The figure shows three views and two pictorial views of one solid part (mm, origin at its lowest corner). Answer the questions. A direction names the side the tool comes from. Round coordinates to 2 decimals unless told otherwise and drop trailing zeros. Write each loop counter-clockwise with the first axis right and the second up, starting at its lowest first coordinate (ties: lowest second). Pieces come first, ordered by that corner, then holes.
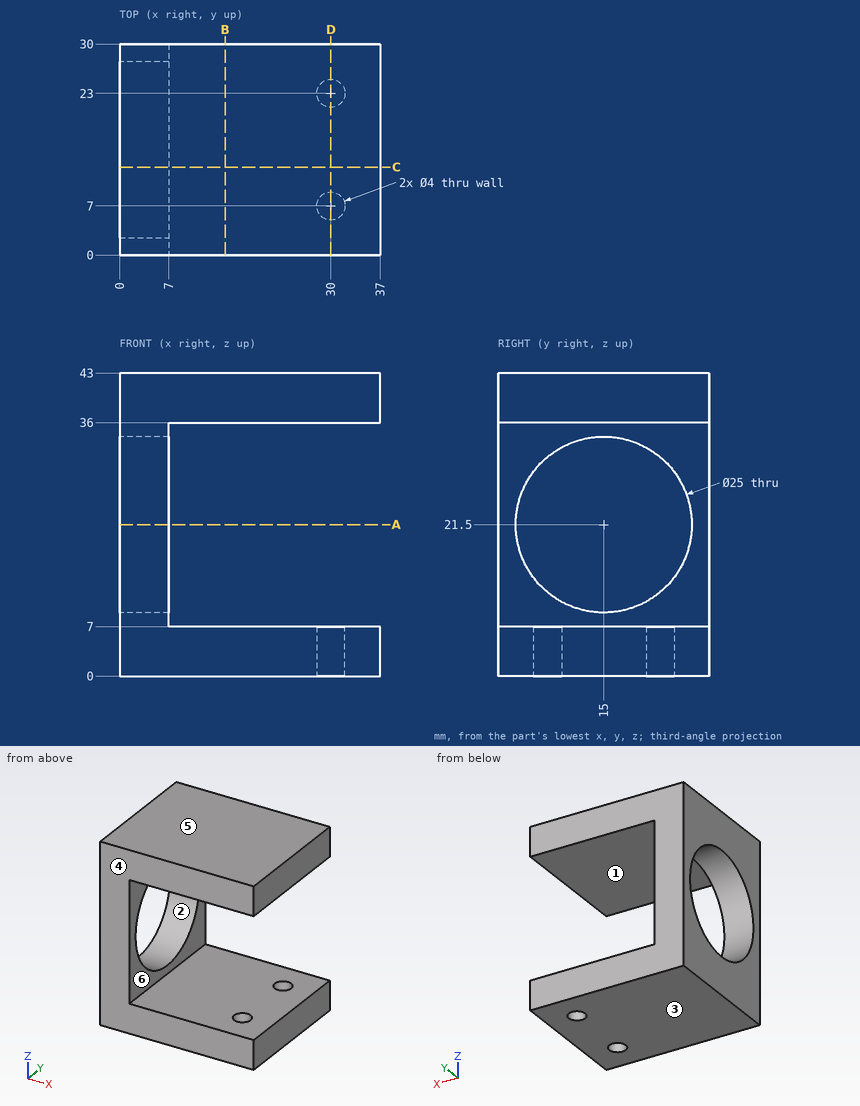
Q1. Straight lines are drawn through the part: probe 1 along Y at (x, z) = (30, 2.75); probe 2 along Z at (x, y) = (21, 18.25); probe 3 along X at (y, z) = (7, 5). For each, find the intervals that lie inside material, in ascending order.
Verdict:
probe 1: y = 0 to 5, 9 to 21, 25 to 30
probe 2: z = 0 to 7, 36 to 43
probe 3: x = 0 to 28, 32 to 37
Q2. Section A-A (z = 21.5) is taken. Determine the outline of the cut face in (x, y), then the cut area to 3 significant figures.
Verdict:
outline: (0, 0) - (7, 0) - (7, 2.5) - (0, 2.5) - close; (0, 27.5) - (7, 27.5) - (7, 30) - (0, 30) - close
area: 35.0 mm2
Q3. Determine the mould class of the marked faces 3, 4, 5 and 6 for opening direction Z: pulls with the +Z half, pulls with the -Z half, needs draft (parallel to the pull), parting line crosses it, or undercut.
Verdict:
face 3: pulls with the -Z half
face 4: needs draft
face 5: pulls with the +Z half
face 6: undercut
Q4. Section B-B (x = 15) is taken. Determine the outline of the cut face in (y, z), then the cut area to 3 significant figures.
Verdict:
outline: (0, 0) - (30, 0) - (30, 7) - (0, 7) - close; (0, 36) - (30, 36) - (30, 43) - (0, 43) - close
area: 420 mm2
Q5. Which of the six approach directions +Z, -Z, +X, -X, +Y, -Y give full straight-line access (tool end or side, diameter ignored) to the marked faces 1 and 2?
Verdict:
face 1: +X, +Y, -Y
face 2: +X, -X
Q6. Section C-C (y = 12.5) is taken. Determine the outline of the cut face in (x, z), then the cut area to 3 significant figures.
Verdict:
outline: (0, 0) - (37, 0) - (37, 7) - (7, 7) - (7, 9.25) - (0, 9.25) - close; (0, 33.75) - (7, 33.75) - (7, 36) - (37, 36) - (37, 43) - (0, 43) - close
area: 550 mm2
Q7. Section D-D (x = 30) is taken. Determine the outline of the cut face in (y, z).
Verdict:
outline: (0, 0) - (5, 0) - (5, 7) - (0, 7) - close; (0, 36) - (30, 36) - (30, 43) - (0, 43) - close; (9, 0) - (21, 0) - (21, 7) - (9, 7) - close; (25, 0) - (30, 0) - (30, 7) - (25, 7) - close
